Part model, mm, in its own coordinate system. A direction names the side the tool comes from. Round coordinates to 2 decimals unless told otherwise and drop trailing zeros. Write each loop counter-clockwise with the first axis right and the second up, starting at its lowest first coordinate (ties: lowest second). Pieces come first, ordered by that corner, then holes. Notation, with made-up numbers: (28.25, 51.5) -> (73.25, 51.5) arc R9 ccw to (73.25, 60.5) -> close; hole circle Ø6 at (55, 72). An arc over 180 degrees is marked (long way). Use CSV: the item, a comma, the result in double quotes. Start each with the question number.
(1) Saw through at C-C (z = 2.4). Count the separate pieces of the cut face and the enclosed holes in it, plus the area to 3 significant figures.
(2) Saw through at B-B (y = -47). Give the cut face in (x, z) (3 decimals), plus the area to 3 significant figures.
(3) Probe line 1 (X direction, y = -6, z = 2.75); line 2 (Y direction, x = 18.5, z = 0.2); line 3 (X direction, y = -44, z = 1.45). List the from-to ranges inside material, lowest first. Write a range as [from, to].
(4) Saw through at A-A (x = 6). Give the cut face in (y, z) (1 decimal), plus the area to 3 significant figures.
(5) Drop flat-ended pins along their axis: pin 1 (1 mm diameter, centred on y = -20, z = 0.5, fed in from +X); pin 2 (1.5 mm diameter, centred on y = -28, z = 0.5, fed in from +X). Give the stop position or say it passes through.
(6) Saw through at D-D (x = 33). Give the cut face in (y, z) (3 decimals), plus the area to 3 significant figures.
(7) Two-plate mould, pull along Y, no slides. Class faces 1 (the flat face through (45.426, -30.849, 1.565)), 2 (the cylindrical face through (10.973, -58.406, 1.565)), 3 (the flat face through (16.84, -7.653, 1.565)): released by +Y, released by -Y, zero draft, split by the parting line, or undercut.
(8) Which spindle directions (+Z, -Z, +X, -X, +Y, -Y) get a long thin tool onto all of the face, cutting with end or side? Do faces 4 (the cylindrical face through (9.772, -9.684, 1.61)), 5 (the cylindrical face through (41.511, -9.385, 1.565)). Say none if no direction does.
```python
from build123d import *

# Parameters (mm, degrees)
BOSS_EXTRUDE1_DEPTH   = 3.175
FILLET1_R             = 3.175
FILLET2_R             = 12.7
F_2_CLEARANCE_HOLE1_D = 2.7051
F_6_CLEARANCE_HOLE1_D = 4.3053


with BuildPart() as part:
    # Sketch1 → Boss-Extrude1 (new body)
    with BuildSketch(Plane.XY):
        with BuildLine():
            Line((13.363407355, -58.995822037), (35.883167135, -55.446288697))
            Line((35.883167135, -55.446288697), (43.833071408, -55.214709803))
            ThreePointArc((43.833071408, -55.214709803), (47.359348086, -53.495537965), (48.398820761, -49.712724781))
            Line((48.398820761, -49.712724781), (42.367918864, -11.450100102))
            ThreePointArc((42.367918864, -11.450100102), (41.492080159, -9.359050224), (39.748688678, -7.90985418))
            Line((39.748688678, -7.90985418), (29.660979166, -2.997190284))
            ThreePointArc((29.660979166, -2.997190284), (29.377888176, -2.875939169), (29.084381769, -2.78268505))
            Line((29.084381769, -2.78268505), (1.220294786, 4.603508106))
            ThreePointArc((1.220294786, 4.603508106), (-3.993511378, 2.594855125), (-3.710688281, -2.98533059))
            Line((-3.710688281, -2.98533059), (2.546868459, -10.763310872))
            Line((2.546868459, -10.763310872), (9.732790422, -56.353877547))
            ThreePointArc((9.732790422, -56.353877547), (11.000934269, -58.426775179), (13.363407355, -58.995822037))
        make_face()
        Polygon((25.134571201, -6.346026675), (32.452304237, -52.772859253), (16.005351845, -55.365205105), (8.687618809, -8.938372527), align=None, mode=Mode.SUBTRACT)
    extrude(amount=BOSS_EXTRUDE1_DEPTH)

    # Fillet1
    fillet1_edges = [part.edges().sort_by_distance(p)[0] for p in [
        (32.452304237, -52.772859253, 1.5875),
        (25.134571201, -6.346026675, 1.5875),
        (8.687618809, -8.938372527, 1.5875),
        (16.005351845, -55.365205105, 1.5875),
    ]]
    fillet(fillet1_edges, radius=FILLET1_R)

    # Fillet2
    fillet2_edges = [part.edges().sort_by_distance(p)[0] for p in [
        (2.546868459, -10.763310872, 1.5875),
        (35.883167135, -55.446288697, 1.5875),
    ]]
    fillet(fillet2_edges, radius=FILLET2_R)

    # #2 Clearance Hole1 (through all)
    with Locations(Plane.XY.offset(3.175)):
        with Locations((5.551338097, -9.432708748), (28.270851912, -5.851690454), (35.588584948, -52.278523032), (12.869071133, -55.859541326)):
            Hole(F_2_CLEARANCE_HOLE1_D / 2)

    # #6 Clearance Hole1 (through all)
    with Locations(Plane.XY.offset(3.175)):
        with Locations((0, 0), (37.663497797, -12.191604434), (43.694399694, -50.454229113)):
            Hole(F_6_CLEARANCE_HOLE1_D / 2)


solid = part.part
```
Answers:
1,separate pieces,"1"
1,enclosed holes,"8"
1,area,"1,420 mm²"
2,outline,"(8.258, 0) -> (14.687, 0) -> (14.687, 3.175) -> (8.258, 3.175) -> close; (31.542, 0) -> (47.971, 0) -> (47.971, 3.175) -> (31.542, 3.175) -> close"
2,area,"72.6 mm²"
3,line 1,"x = [-1.29, 26.93], [29.62, 35.83]"
3,line 2,"y = [-58.19, -54.91], [-7.39, 0.02]"
3,line 3,"x = [7.79, 14.21], [31.07, 47.5]"
4,outline,"(-32.7, 0) -> (-10.7, 0) -> (-10.7, 3.2) -> (-32.7, 3.2) -> close; (-8.2, 0) -> (3.3, 0) -> (3.3, 3.2) -> (-8.2, 3.2) -> close"
4,area,"106 mm²"
5,pin 1,"stops at x = 43.79"
5,pin 2,"stops at x = 45.09"
6,outline,"(-55.901, 0) -> (-4.623, 0) -> (-4.623, 3.175) -> (-55.901, 3.175) -> close"
6,area,"163 mm²"
7,face 1,"released by +Y"
7,face 2,"released by -Y"
7,face 3,"undercut"
8,face 4,"+Z, -Z"
8,face 5,"+Z, -Z, +X, +Y"
